Autodesk Inventor part; units mm, degrees
ref_plane "YZ Plane" through (0, 0, 0) normal (1, 0, 0) x (0, 1, 0)
ref_plane "XZ Plane" through (0, 0, 0) normal (0, 1, 0) x (-1, 0, 0)
ref_plane "XY Plane" through (0, 0, 0) normal (0, 0, 1) x (1, 0, 0)
sketch "Sketch1" plane through (0, 0, 0) normal (0, 1, 0) x (-1, 0, 0)
  line L0 (-63.5, -12.7) -> (63.5, -12.7)
  line L1 (63.5, -12.7) -> (63.5, 12.7)
  line L2 (63.5, 12.7) -> (-63.5, 12.7)
  line L3 (-63.5, 12.7) -> (-63.5, -12.7)
  line L4 (-63.5, -12.7) -> (63.5, 12.7) construction
  line L5 (63.5, -12.7) -> (-63.5, 12.7) construction
  point P0 (0, 0)
  dimension "d0" = 127
  dimension "d1" = 25.4
extrude "Extrusion1" add sketch "Sketch1" along normal blind 6.35
sketch "Sketch2" plane through (0, 6.35, 0) normal (0, 1, 0) x (1, 0, 0)
  line L0 (-63.5, 12.7) -> (-63.5, -12.7)
  line L1 (63.5, -12.7) -> (63.5, 12.7)
  line L2 (-63.5, 0) -> (-50.8, 0)
  line L3 (-63.5, 0) -> (-50.8, 0) construction
  line L4 (63.5, 0) -> (50.8, 0)
  line L5 (63.5, 0) -> (76.2, 0) construction
  circle A0 centre (-50.8, 0) radius 3.175
  circle A1 centre (50.8, 0) radius 3.175
  point P0 (0, 0)
  dimension "d4" = 12.7
  dimension "d5" = 0
  dimension "d6" = 12.7
  dimension "d7" = 180
  dimension "d8" = 6.35
  dimension "d9" = 6.35
extrude "Extrusion2" cut sketch "Sketch2" against normal blind 6.35
sketch "Sketch3" plane through (0, 6.35, 0) normal (0, 1, 0) x (1, 0, 0)
  circle A0 centre (0, 0) radius 6.35
  line L0 (-6.35, 0) -> (-3.175, 5.4993)
  line L1 (-3.175, 5.4993) -> (3.175, 5.4993)
  line L2 (3.175, 5.4993) -> (6.35, 0)
  line L3 (6.35, 0) -> (3.175, -5.4993)
  line L4 (3.175, -5.4993) -> (-3.175, -5.4993)
  line L5 (-3.175, -5.4993) -> (-6.35, 0)
  dimension "d12" = 12.7
extrude "Extrusion3" cut sketch "Sketch3" against normal blind 25.4 contours L3 L4 L5 L0 L1 L2
properties part number "ArmPlate"
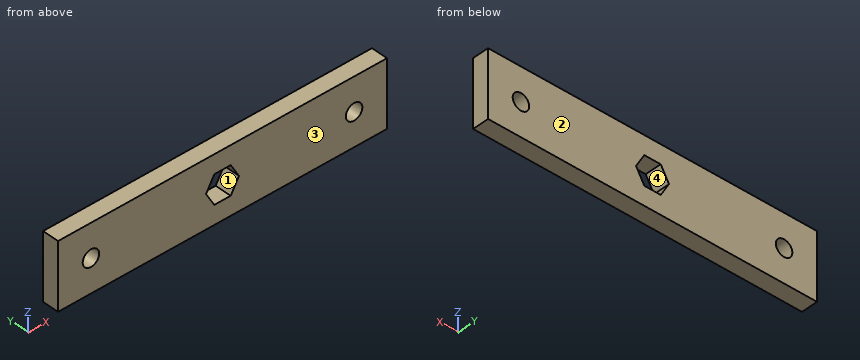
Can you work these out from the model? Positions are in its coordinate system, mm. Face numbers are marked on the shaded views. A direction names the side the tool comes from. Give positions to 0.01 mm unless a question says otherwise; leave off trailing zeros. Loops run counter-clockwise (first coordinate to the right, second up) from the corner with the lowest first, then second, coordinate; pieces in that order, holes last. Notation, with made-up numbers: (67, -29.5) - (79, -29.5) arc R20 ccw to (79, -7.5) - close; hole circle Ø7 at (56.5, 7.5). An arc over 180 degrees is marked (long way). One line per item, written item: value.
(1) If we section it at A-A, the plane x = 50.8: List the corners of the cut face in (y, z) for me (3 decimals).
Verdict:
outline: (0, -12.7) - (6.35, -12.7) - (6.35, -3.175) - (0, -3.175) - close; (0, 3.175) - (6.35, 3.175) - (6.35, 12.7) - (0, 12.7) - close
(2) If we mould it in two halves opening along Z, with no side actions, what happens to the marked faces 1 and 2? For each: released by +Z, released by -Z, zero draft, split by the parting line, or undercut.
Verdict:
face 1: undercut
face 2: zero draft
(3) On a 3-axis mill with a long thin cutter (end or side, diameter ignored), from which of +Z, -Z, +X, -X, +Y, -Y can I reach the whole of each face in a straight line? I mean the marked faces 3 and 4. Say none if no direction works.
Verdict:
face 3: +Z, -Z, +X, -X, -Y
face 4: +Y, -Y
(4) I'm going to push a flat-ended pin straight in: pin 1 (5.5 mm diameter, centred on x = 50.8, z = 0, fed in from +Y). Where does the tip first touch, or does it pass through?
Verdict:
pin 1: through
(5) If we section it at B-B, the plane y = 1.25: List the corners of the cut face in (x, z) for me (3 decimals), plus the area to 3 significant figures.
Verdict:
outline: (-63.5, -12.7) - (63.5, -12.7) - (63.5, 12.7) - (-63.5, 12.7) - close; hole circle Ø6.35 at (-50.8, 0); hole (-6.35, 0) - (-3.175, -5.499) - (3.175, -5.499) - (6.35, 0) - (3.175, 5.499) - (-3.175, 5.499) - close; hole circle Ø6.35 at (50.8, 0)
area: 3,060 mm^2
(6) I need wall thicknesses on line 1 along X through (y, z) = (1.5, 0) (3 decimals); line 2 along X through (y, z) = (6, 2.5); line 3 along Z through (x, y) = (50.8, 4) (3 decimals). Which ranges of each line are inside material? Lowest first, please.
Verdict:
line 1: -63.5 to -53.975, -47.625 to -6.35, 6.35 to 47.625, 53.975 to 63.5
line 2: -63.5 to -52.76, -48.84 to -4.91, 4.91 to 48.84, 52.76 to 63.5
line 3: -12.7 to -3.175, 3.175 to 12.7
(7) If we section it at C-C, the plane z = 1.5: List the corners of the cut face in (x, y) for me, plus the area to 3 significant figures.
Verdict:
outline: (-63.5, 0) - (-53.6, 0) - (-53.6, 6.35) - (-63.5, 6.35) - close; (-48, 0) - (-5.48, 0) - (-5.48, 6.35) - (-48, 6.35) - close; (5.48, 0) - (48, 0) - (48, 6.35) - (5.48, 6.35) - close; (53.6, 0) - (63.5, 0) - (63.5, 6.35) - (53.6, 6.35) - close
area: 666 mm^2
